Autodesk Inventor part; units mm, degrees
ref_plane "YZ Plane" through (0, 0, 0) normal (1, 0, 0) x (0, 1, 0)
ref_plane "XZ Plane" through (0, 0, 0) normal (0, 1, 0) x (-1, 0, 0)
ref_plane "XY Plane" through (0, 0, 0) normal (0, 0, 1) x (1, 0, 0)
sketch "Boceto1" plane through (0, 0, 0) normal (1, 0, 0) x (0, 1, 0)
  line L0 (0, 0) -> (105, 0)
  line L1 (105, 0) -> (105, -85)
  line L2 (105, -85) -> (0, -85)
  line L3 (0, -85) -> (0, 0)
  line L4 (110, 5) -> (-5, 5)
  line L5 (-5, 5) -> (-5, -90)
  line L6 (-5, -90) -> (110, -90)
  line L7 (110, -90) -> (110, 5)
  point P0 (105, -42.5)
  dimension "d0" = 85
  dimension "d1" = 105
  dimension "d2" = 5
  dimension "d3" = 5
  dimension "d4" = 5
  dimension "d5" = 5
extrude "Extrusión1" add sketch "Boceto1" along normal blind 30
extrude "Extrusión2" add sketch "Boceto1" along normal blind 5 contours L0 L1 L2 L3
sketch "Boceto2" plane through (0, -5, -90) normal (0, -1, 0) x (1, 0, 0)
  line L0 (0, 0) -> (30, 0)
  line L1 (30, 0) -> (30, 2)
  line L2 (30, 0) -> (30, 95)
  line L3 (28, 2) -> (25, 4)
  line L4 (25, 4) -> (25, 0)
  line L5 (25, 0) -> (30, 0)
  line L6 (30, 2) -> (28, 2)
  line L7 (37.2923, 47.5) -> (-11.4995, 47.5) construction
  line L8 (30, 95) -> (30, 93)
  line L9 (28, 93) -> (25, 91)
  line L10 (25, 91) -> (25, 95)
  line L11 (25, 95) -> (30, 95)
  line L12 (30, 93) -> (28, 93)
  point P0 (0, 90)
  point P1 (30, 47.5)
  point P2 (25, 0)
  dimension "d10" = 2
  dimension "d11" = 2
  dimension "d12" = 4
  dimension "d13" = 5
  dimension "d14" = 0
extrude "Extrusión3" cut sketch "Boceto2" against normal blind 110
properties part number "carcasa_pcb"
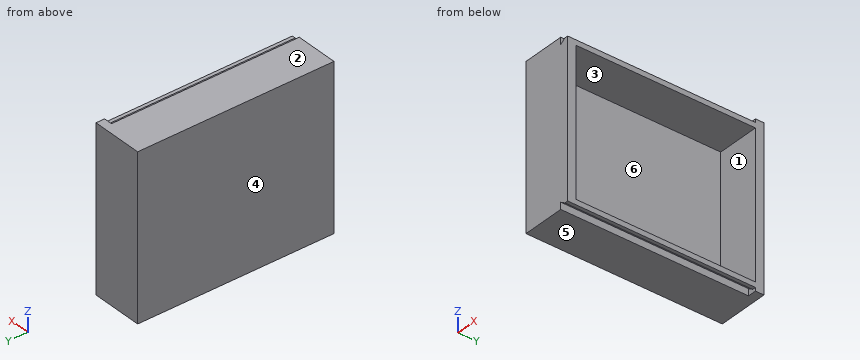
Source: CAD feature listing. Evaluate the final solid. Frame: model axes, mm. Face numbers are marked on the shaded views. A direction names the side the tool comes from. Round coordinates to 2 decimals unless told otherwise and drop trailing zeros. Order: outer loops, then holes, each group sorted by start corner. A loop starts at its lowest first (then second) coordinate and runs counter-clockwise, first axis right, second up. Notation, with made-up numbers: (20.25, 23) -> (62.25, 23) arc R28 cw to (62.25, 46) -> close; hole circle Ø8 at (-8.5, 32). An arc over 180 degrees is marked (long way). One line per item, written item: value. Start each with the question number.
Q1. Pin query (flat end, axial travel): pin 1 (5 mm diameter, centred on y = 71, z = -8.5, fed in from +X); pin 2 (3 mm diameter, centred on x = 27, z = 3, fed in from -Y); pin 3 (1.6 mm diameter, centred on x = 28.5, y = 72, fed in from +Z); pin 4 (2 mm diameter, centred on x = 29, y = 74.5, fed in from -Z). Return the tip coordinate at first contact, or that it passes through.
Q2. Material intervals for probe 1 along Y at (x, z) = (14.25, -63); probe 2 along Z at (x, y) = (8.5, 44.5); probe 3 along X at (y, z) = (15, -31), sorted ascending.
Q3. Section query D-D (x = 17.25). Return the cut outline in (y, z).
Q4. Access query for the marked faces 5 and 6. Directions: +Z, -Z, +X, -X, +Y, -Y. A direction counts if a zero-diameter tool reaches every point of the face in a straight line with its end or side. Return the directions, or none.
Q5. Draft query along Z for the marked faces 1, 2, 3 and 4. Return one class per face: pulls with the +Z half, pulls with the -Z half, needs draft (parallel to the pull), parting line crosses it, or undercut.
Q6. Section query B-B (z = -6.5). Return the cut outline in (x, y), plus the area to 3 significant figures.
Q7. Section query A-A (x = 26.5). Return the cut outline in (y, z).
Q8. Section query C-C (y = 51). Return the cut outline in (x, z), plus the area to 3 significant figures.
Findings below:
1. pin 1: x = 5
1. pin 2: y = -5
1. pin 3: z = 3
1. pin 4: z = -88
2. probe 1: -5 to 0, 105 to 110
2. probe 2: -90 to -85, 0 to 5
2. probe 3: 0 to 5
3. outline: (-5, -90) -> (110, -90) -> (110, 5) -> (-5, 5) -> close; hole (0, -85) -> (105, -85) -> (105, 0) -> (0, 0) -> close
4. face 5: -Z, +X, -X, +Y, -Y
4. face 6: +X
5. face 1: undercut
5. face 2: pulls with the +Z half
5. face 3: undercut
5. face 4: needs draft
6. outline: (0, -5) -> (30, -5) -> (30, 0) -> (5, 0) -> (5, 105) -> (30, 105) -> (30, 110) -> (0, 110) -> close
6. area: 825 mm²
7. outline: (-5, -87) -> (105, -87) -> (105, -90) -> (110, -90) -> (110, 5) -> (105, 5) -> (105, 2) -> (-5, 2) -> close; hole (0, -85) -> (105, -85) -> (105, 0) -> (0, 0) -> close
8. outline: (0, -90) -> (25, -90) -> (25, -86) -> (28, -88) -> (30, -88) -> (30, -85) -> (5, -85) -> (5, 0) -> (30, 0) -> (30, 3) -> (28, 3) -> (25, 1) -> (25, 5) -> (0, 5) -> close
8. area: 699 mm²
